Model file for the job. Use its own axes, mm. A direction names the side the tool comes from. Coordinates: 2 decimals unless noted, no trailing zeros. Write each loop counter-clockwise with the first axis right and the second up, starting at its lowest first coordinate (ties: lowest second). Pieces come first, ordered by that corner, then holes. Notation, with made-up numbers: (13.5, 2.5) - (27.5, 2.5) arc R22 ccw to (27.5, 40.5) - close; hole circle Ø10 at (17, 47.5). An arc over 180 degrees is marked (long way). Put each result on its own line as item: value. Start each with the question number.
1. Saw through at B-B, the plane x = 0. Give the number of separate pieces and of enclosed holes in the cut face, plus the area to 3 significant figures.
2. Saw through at C-C, the plane y = 346. Write the cut outline in (x, z), plus the area to 3 significant figures.
3. Drill centre lines: L1, parallel to Z at x = 7.75, y = 337; L2, parallel to X at y = 260, z = 18.5; L3, parallel to X at y = 260, z = 5. Where is each one in solid material? Low to high. Write a range as from..to.
4. Drop flat-ended pins along their axis: P1, Ø10, axis at x = 0, y = 380, coming from the +Z side; P2, Ø10, axis at x = 0, y = 200, coming from the -Z side; P3, Ø3.5, axis at y = 156, z = 11.5, coming from the +X side; P4, Ø3.5, axis at y = 142.5, z = 11.5, coming from the -X side. Give the stop position or say it passes through.
5. Pull direction X, two halves, no side cores. Call faces 1 (the face through (0, 400, 11)), 2 (the face through (-1.05, 316.66, 6.41)): released by +X, released by -X, zero draft, split by the parting line, or undercut.
6. Which spindle directions (+Z, -Z, +X, -X, +Y, -Y) get a long thin tool onto all of the face, cutting with end or side? Do faces 3 (the face through (4, 320, 13)), 4 (the face through (-1.05, 256.66, 6.41)). Say none if no direction does.
Autodesk Fusion 360 part; units mm, degrees
sketch "Sketch2" plane through (0, 0, 0) normal (0, 1, 0) x (1, 0, 0)
  line L0 (0, 0) -> (-10, 0)
  line L1 (-10, 0) -> (-11.5, -1.5)
  line L2 (-11.5, -1.5) -> (-11.5, -6.199)
  line L3 (-11.5, -6.199) -> (-7.7, -9.999)
  line L4 (-7.7, -9.999) -> (-7.7, -13.38)
  line L5 (-11.5, -17.08) -> (-11.5, -19.109)
  line L6 (-8.5085, -22) -> (0, -22)
  line L7 (0, -37) -> (0, 7) construction
  arc A0 (-8.9292, -21.5934) -> (-11.2845, -19.3172) centre (-11.447, -21.842) ccw
  line L8 (-11.5, -19.109) -> (-11.2845, -19.3172)
  line L9 (-8.9292, -21.5934) -> (-8.5085, -22)
  arc A1 (-11.2972, -16.8826) -> (-8.9263, -14.5741) centre (-11.447, -14.357) ccw
  line L10 (-7.7, -13.38) -> (-8.9263, -14.5741)
  line L11 (-11.2972, -16.8826) -> (-11.5, -17.08)
  line L12 (0, 0) -> (10, 0)
  line L13 (10, 0) -> (11.5, -1.5)
  line L14 (11.5, -1.5) -> (11.5, -6.199)
  line L15 (11.5, -6.199) -> (7.7, -9.999)
  line L16 (7.7, -9.999) -> (7.7, -13.38)
  line L17 (7.7, -13.38) -> (8.9263, -14.5741)
  arc A2 (8.9263, -14.5741) -> (11.2972, -16.8826) centre (11.447, -14.357) ccw
  line L18 (11.2972, -16.8826) -> (11.5, -17.08)
  line L19 (11.5, -17.08) -> (11.5, -19.109)
  line L20 (11.5, -19.109) -> (11.2845, -19.3172)
  arc A3 (11.2845, -19.3172) -> (8.9292, -21.5934) centre (11.447, -21.842) ccw
  line L21 (8.9292, -21.5934) -> (8.5085, -22)
  line L22 (8.5085, -22) -> (0, -22)
  dimension "d29" = 10
  dimension "d30" = 1.5
  dimension "d31" = 1.5
  dimension "d32" = 3.381
  dimension "d33" = 3.7
  dimension "d34" = 22
  dimension "d35" = 3.8
  dimension "d36" = 3.8
  dimension "d38" = 8.5085
  dimension "d39" = 2.029
  dimension "d40" = 2.891
  dimension "d42" = 11.447
  dimension "d43" = 0.158
  dimension "d46" = 2.53
  dimension "d47" = 2.53
  dimension "d48" = 7.485
extrude "Extrude2" add sketch "Sketch2" along normal blind 400
hole "Hole4" at (0, 80, 22) direction (0, 0, -1) diameter 7 depth 22 tip angle 118 counterbore diameter 11 counterbore depth 9
pattern_linear "R-Pattern4" count 7 spacing 60 along (0, 1, 0) of "Hole4"
equation "RailLength = 400 mm"
equation "RailHoleSpacing = 60 mm"
equation "RailFirstHoleOffset = ( RailLength - ( ( RailNumberOfHoles - 1 ) * RailHoleSpacing ) ) / 2"
equation "d53 = RailLength"
equation "d96 = RailHoleSpacing"
Final values:
1. separate pieces: 7
1. enclosed holes: 0
1. area: 7,660 mm²
2. outline: (-11.5, 1.5) - (-10, 0) - (10, 0) - (11.5, 1.5) - (11.5, 6.2) - (7.7, 10) - (7.7, 13.38) - (8.93, 14.57) arc R2.53 cw to (11.3, 16.88) - (11.5, 17.08) - (11.5, 19.11) - (11.28, 19.32) arc R2.53 cw to (8.93, 21.59) - (8.51, 22) - (-8.51, 22) - (-8.93, 21.59) arc R2.53 cw to (-11.28, 19.32) - (-11.5, 19.11) - (-11.5, 17.08) - (-11.3, 16.88) arc R2.53 cw to (-8.93, 14.57) - (-7.7, 13.38) - (-7.7, 10) - (-11.5, 6.2) - close
2. area: 435 mm²
3. L1: z = 0..9.95, 13.43..22
3. L2: x = -11.5..-5.5, 5.5..11.5
3. L3: x = -11.5..-3.5, 3.5..11.5
4. P1: stops at z = 13
4. P2: stops at z = 0
4. P3: stops at x = 7.95
4. P4: stops at x = -7.95
5. face 1: zero draft
5. face 2: undercut
6. face 3: +Z
6. face 4: +Z, -Z
